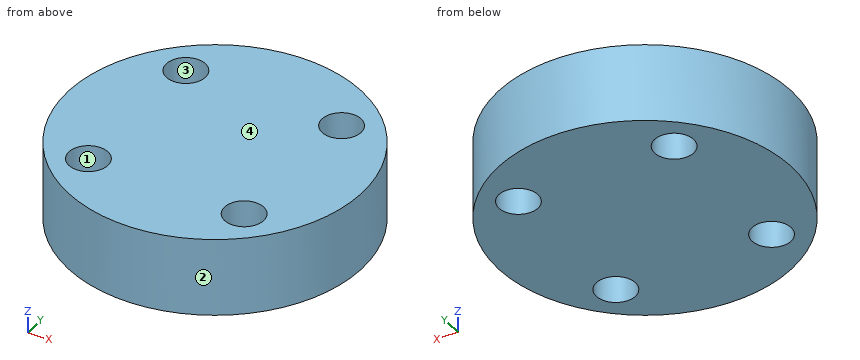
```python
from build123d import *

# Parameters (mm, degrees)
CYLINDER1384_R     = 1
CYLINDER1384_DEPTH = 20
CYLINDER1389_R     = 1
CYLINDER1389_DEPTH = 20
CYLINDER1379_R     = 1
CYLINDER1379_DEPTH = 20
CYLINDER1391_R     = 1
CYLINDER1391_DEPTH = 20
CYLINDER1376_R     = 7.5
CYLINDER1376_DEPTH = 4


with BuildPart() as obj1:
    # Cylinder1384 → Cylinder1384 (new body)
    with BuildSketch(Plane(origin=(4, -4, -88), x_dir=(0, 1, 0), z_dir=(0, 0, 1))):
        Circle(CYLINDER1384_R)
    extrude(amount=CYLINDER1384_DEPTH)


with BuildPart() as obj2:
    # Cylinder1389 → Cylinder1389 (new body)
    with BuildSketch(Plane(origin=(4, 4, -88), x_dir=(-1, 0, 0), z_dir=(0, 0, 1))):
        Circle(CYLINDER1389_R)
    extrude(amount=CYLINDER1389_DEPTH)


with BuildPart() as obj3:
    # Cylinder1379 → Cylinder1379 (new body)
    with BuildSketch(Plane(origin=(-4, 4, -88), x_dir=(0, -1, 0), z_dir=(0, 0, 1))):
        Circle(CYLINDER1379_R)
    extrude(amount=CYLINDER1379_DEPTH)


with BuildPart() as compound959:
    # Cylinder1391 → Cylinder1391 (new body)
    with BuildSketch(Plane(origin=(-4, -4, -88), x_dir=(1, 0, 0), z_dir=(0, 0, 1))):
        Circle(CYLINDER1391_R)
    extrude(amount=CYLINDER1391_DEPTH)

    # Compound959: union obj1, obj2, obj3
    add(obj1.part)
    add(obj2.part)
    add(obj3.part)


with BuildPart() as compound959_1:
    # Compound959 placement: moved
    add(compound959.part.moved(Location((0, 0, 91))))


with BuildPart() as cut499:
    # Cylinder1376 → Cylinder1376 (new body)
    with BuildSketch(Plane.XY.offset(15)):
        Circle(CYLINDER1376_R)
    extrude(amount=CYLINDER1376_DEPTH)

    # Cut499: cut Compound959
    add(compound959_1.part, mode=Mode.SUBTRACT)


solid = cut499.part
```
Read the model definition and answer for the solid it produces. Units are mm, in the model's axes. Face numbers are marked on the shaded views. Coordinates: 2 decimals unless noted, no trailing zeros. Loops run counter-clockwise (first coordinate to the right, second up) from the corner with the lowest first, then second, coordinate; pieces in that order, holes last. Notation, with made-up numbers: (10.5, -21) - (62.5, -21) arc R26 ccw to (62.5, -6) - close; hole circle Ø5 at (77.25, 82.25). An arc over 180 degrees is marked (long way). Answer in a Markdown table with one row per item.
1. Straight lines are drawn through the part: line 1 (X direction, y = -4, z = 18.15); line 2 (Y direction, x = -4.5, z = 15.2). For each, find the intervals that lie inside material, in ascending order.
Conclusion:
| item | result |
|---|---|
| line 1 | x = -6.34 to -5, -3 to 3, 5 to 6.34 |
| line 2 | y = -6 to -4.87, -3.13 to 3.13, 4.87 to 6 |
2. Determine the mould class of the marked faces 1, 2, 3 and 4 for opening direction X: +X half, -X half, draft (parallel to the pull), parting line (faces both ways), or undercut.
Conclusion:
| item | result |
|---|---|
| face 1 | undercut |
| face 2 | parting line |
| face 3 | undercut |
| face 4 | draft |
3. Find section A-A, the plane y = 4. Write down the section's boundary in (x, z).
Conclusion:
| item | result |
|---|---|
| outline | (-6.34, 15) - (-5, 15) - (-5, 19) - (-6.34, 19) - close; (-3, 15) - (3, 15) - (3, 19) - (-3, 19) - close; (5, 15) - (6.34, 15) - (6.34, 19) - (5, 19) - close |
4. Find section D-D, the plane y = -1.5. Write down the section's boundary in (x, z), then the cut area to 3 significant figures.
Conclusion:
| item | result |
|---|---|
| outline | (-7.35, 15) - (7.35, 15) - (7.35, 19) - (-7.35, 19) - close |
| area | 58.8 mm² |
5. Find section B-B, the plane z = 17.4. Write down the section's boundary in (x, y), then the cut area to 3 significant figures.
Conclusion:
| item | result |
|---|---|
| outline | circle Ø15 at (0, 0); hole circle Ø2 at (-4, -4); hole circle Ø2 at (-4, 4); hole circle Ø2 at (4, -4); hole circle Ø2 at (4, 4) |
| area | 164 mm² |
6. Given pin 1 (1.2 mm diameter, centred on x = 4, y = 4, fed in from -Z); pin 2 (1 mm diameter, centred on y = -2, z = 15.5, fed in from -X); pin 3 (2 mm diameter, centred on y = -6, z = 17.5, fed in from -X), each flat-ended and moving along its own axis, determine where each tip first touches the part or whether it passes through.
Conclusion:
| item | result |
|---|---|
| pin 1 | passes through |
| pin 2 | stops at x = -7.35 |
| pin 3 | stops at x = -5.59 |
